Geometry check sheet. Reference: the model listing, model coordinates, mm. A direction names the side the tool comes from. Give positions to 0.01 mm unless a question says otherwise; leave off trailing zeros. Loops run counter-clockwise (first coordinate to the right, second up) from the corner with the lowest first, then second, coordinate; pieces in that order, holes last. Notation, with made-up numbers: (-9.5, -30.5) -> (10.5, -30.5) arc R20 cw to (10.5, -17.5) -> close; hole circle Ø10 at (77.25, -26). An arc over 180 degrees is marked (long way). Answer in a Markdown table with one row per item. Add a question column.
```python
from build123d import *

# Parameters (mm, degrees)
SKETCH_W        = 174
SKETCH_H        = 19
PAD_DEPTH       = 8.55
SKETCH001_W     = 170
SKETCH001_H     = 16
POCKET_DEPTH    = 7.3
SKETCH002_R     = 1.1
HOLE_DEPTH      = 174.001
CHAMFER_SIZE    = 1.4
SKETCH003_W     = 174
SKETCH003_H     = 1.5
PAD001_DEPTH    = 3.45
SKETCH004_W     = 174
SKETCH004_H     = 5
PAD002_DEPTH    = 5
FILLET_R        = 1
SKETCH005_W     = 5
SKETCH005_H     = 10.149898
SKETCH005_H_2   = 10.668564
SKETCH005_H_3   = 8.55
SKETCH005_H_4   = 9.73434
SKETCH005_H_5   = 10.175496
POCKET001_DEPTH = 20


with BuildPart() as part:
    # Sketch → Pad (new body)
    with BuildSketch(Plane.XY):
        with Locations((0, -0.5)):
            Rectangle(SKETCH_W, SKETCH_H)
    extrude(amount=PAD_DEPTH)

    # Sketch001 → Pocket (cut)
    with BuildSketch(Plane(origin=(0, 0, 0), x_dir=(1, 0, 0), z_dir=(0, 0, -1))):
        with Locations((0, 0.5)):
            Rectangle(SKETCH001_W, SKETCH001_H)
    extrude(amount=-POCKET_DEPTH, mode=Mode.SUBTRACT)

    # Sketch002 (on Face3 of Pocket) → Hole (cut, through all)
    with BuildSketch(Plane.YZ.offset(87)):
        with Locations((5, 4.75)):
            Circle(SKETCH002_R)
    extrude(amount=-HOLE_DEPTH, mode=Mode.SUBTRACT)

    # Chamfer
    chamfer_edges = [part.edges().sort_by_distance(p)[0] for p in [
        (0, 9, 0),
    ]]
    chamfer(chamfer_edges, length=CHAMFER_SIZE)

    # Sketch003 (on Face6 of Chamfer) → Pad001 (join)
    with BuildSketch(Plane(origin=(0, 0, 0), x_dir=(1, 0, 0), z_dir=(0, 0, -1))):
        with Locations((0, 9.25)):
            Rectangle(SKETCH003_W, SKETCH003_H)
    extrude(amount=PAD001_DEPTH)

    # Sketch004 (on Face8 of Pad001) → Pad002 (join)
    with BuildSketch(Plane.XZ.offset(10)):
        with Locations((0, 6.05)):
            Rectangle(SKETCH004_W, SKETCH004_H)
    extrude(amount=PAD002_DEPTH)

    # Fillet
    fillet_edges = [part.edges().sort_by_distance(p)[0] for p in [
        (-87, -12.5, 8.55),
        (-87, -0.5, 8.55),
        (87, -0.5, 8.55),
        (87, -12.5, 8.55),
        (0, 9, 8.55),
        (0, -15, 8.55),
        (87, -15, 6.05),
        (0, -15, 3.55),
        (-87, -15, 6.05),
    ]]
    fillet(fillet_edges, radius=FILLET_R)

    # Sketch005 (on Face12 of Fillet) → Pocket001 (cut)
    with BuildSketch(Plane.XY.offset(8.55)):
        with Locations((-7.3085, 11.524949)):
            Rectangle(SKETCH005_W, SKETCH005_H)
        with Locations((7.3085, 11.784282)):
            Rectangle(SKETCH005_W, SKETCH005_H_2)
        with Locations((-21.9255, 10.725)):
            Rectangle(SKETCH005_W, SKETCH005_H_3)
        with Locations((-36.5425, 10.725)):
            Rectangle(SKETCH005_W, SKETCH005_H_3)
        with Locations((-51.1595, 10.725)):
            Rectangle(SKETCH005_W, SKETCH005_H_3)
        with Locations((-65.7765, 10.725)):
            Rectangle(SKETCH005_W, SKETCH005_H_3)
        with Locations((-80.3935, 10.725)):
            Rectangle(SKETCH005_W, SKETCH005_H_3)
        with Locations((21.9255, 11.31717)):
            Rectangle(SKETCH005_W, SKETCH005_H_4)
        with Locations((36.5425, 11.537748)):
            Rectangle(SKETCH005_W, SKETCH005_H_5)
        with Locations((51.1595, 10.725)):
            Rectangle(SKETCH005_W, SKETCH005_H_3)
        with Locations((65.7765, 10.725)):
            Rectangle(SKETCH005_W, SKETCH005_H_3)
        with Locations((80.3935, 10.725)):
            Rectangle(SKETCH005_W, SKETCH005_H_3)
    extrude(amount=-POCKET001_DEPTH, mode=Mode.SUBTRACT)


with BuildPart() as part_1:
    # Body placement: moved
    add(part.part.moved(Location((0, -5, -4.75))))


solid = part_1.part
```
1. Release check for a two-part mould opening along X. For faces 1 (the face through (-87, -7, 0)), 2 (the face through (-1, -13.5, -3)), 3 (the face through (58, 4, 0)) record: released by +X, released by -X, zero draft, split by the parting line, or undercut.
2. Gauge pin test, flat ends, axial feed: pin 1 Ø8 at (x, y) = (-14, -6.5) entering from -Z; pin 2 Ø2 at (x, z) = (-43.5, -2.5) entering from -Y; pin 3 Ø6 at (x, z) = (6, 2.5) entering from +Y; pin 4 Ø1.4 at (x, z) = (7, 3) entering from +Y. Record the tip position at first contact, or that the pin passes through.
3. Material ranges on L1, parallel to Y at x = -34, z = -2.25; L2, parallel to X at y = 2.25, z = -3.5; L3, parallel to Y at x = 39.5, z = 0.25, recorded low to high. Write a range as from..to.
4. Access from +Z, -Z, +X, -X, +Y, -Y to the whole of each face (thin tool, end or side, straight path). Record for faces 4 (the face through (-59, 4, 0)), 5 (the face through (-15, 2.5, -1)), 6 (the face through (-1, -15, -5)), 7 (the face through (-86, -5, -4.75)).
5. Sectioned sample at C-C (x = -22.5). Enter the section's corners in (y, z).
6. Sectioned sample at B-B (y = -5.25). Enter the section's corners in (x, z).
7. Sectioned sample at A-A (x = 27.5). Enter the section's corners in (y, z), plus the area to 3 significant figures.
Response:
| question | item | result |
|---|---|---|
| 1 | face 1 | released by -X |
| 1 | face 2 | undercut |
| 1 | face 3 | zero draft |
| 2 | pin 1 | stops at z = 2.55 |
| 2 | pin 2 | stops at y = -15 |
| 2 | pin 3 | stops at y = 4 |
| 2 | pin 4 | stops at y = 1.45 |
| 3 | L1 | y = -15..-13.5, 2.5..4 |
| 3 | L2 | x = -87..-85, 85..87 |
| 3 | L3 | y = -20..-13.5, 2.5..4 |
| 4 | face 4 | +Z, -Z, +X, -X, +Y |
| 4 | face 5 | -Z |
| 4 | face 6 | -Z, +X, -X, -Y |
| 4 | face 7 | -Z, +X, -X, +Y |
| 5 | outline | (-20, -0.2) arc R1 ccw to (-19, -1.2) -> (-15, -1.2) -> (-15, -8.2) -> (-13.5, -8.2) -> (-13.5, 2.55) -> (1.45, 2.55) -> (1.45, 3.8) -> (-19, 3.8) arc R1 ccw to (-20, 2.8) -> close |
| 6 | outline | (-87, -4.75) -> (-85, -4.75) -> (-85, 2.55) -> (85, 2.55) -> (85, -4.75) -> (87, -4.75) -> (87, 2.8) arc R1 ccw to (86, 3.8) -> (-86, 3.8) arc R1 ccw to (-87, 2.8) -> close |
| 7 | outline | (-20, -0.2) arc R1 ccw to (-19, -1.2) -> (-15, -1.2) -> (-15, -8.2) -> (-13.5, -8.2) -> (-13.5, 2.55) -> (2.5, 2.55) -> (2.5, -4.75) -> (2.6, -4.75) -> (4, -3.35) -> (4, 2.8) arc R1 ccw to (3, 3.8) -> (-19, 3.8) arc R1 ccw to (-20, 2.8) -> close |
| 7 | area | 74.2 mm2 |
